Build history of the part. All positions in model axes, mm. Round coordinates to 2 decimals unless told otherwise and drop trailing zeros. Write each loop counter-clockwise with the first axis right and the second up, starting at its lowest first coordinate (ties: lowest second). Pieces come first, ordered by that corner, then holes.
from build123d import *

# Parameters (mm, degrees)
BOSS_EXTRUDE1_DEPTH = 14
CHAMFER1_SIZE       = 2


with BuildPart() as part:
    # Sketch1 → Boss-Extrude1 (new body)
    with BuildSketch(Plane.XY):
        Polygon((4, 3), (61, 3), (53, 31), (12, 38), align=None)
    extrude(amount=BOSS_EXTRUDE1_DEPTH)

    # Chamfer1
    chamfer1_edges = [part.edges().sort_by_distance(p)[0] for p in [
        (53, 31, 7),
    ]]
    chamfer(chamfer1_edges, length=CHAMFER1_SIZE)


solid = part.part
1) Wall check: L1, parallel to X at y = 11, z = 2.25; L2, parallel to X at y = 15.5, z = 2; L3, parallel to Y at x = 33, z = 4. Give the ranges that are in metal, low to high.
Results:
L1: x = 5.83 to 58.71
L2: x = 6.86 to 57.43
L3: y = 3 to 34.41
2) Slice it at C-C (y = 11). Write the cut outline in (x, z), plus the area to 3 significant figures.
Results:
outline: (5.83, 0) - (58.71, 0) - (58.71, 14) - (5.83, 14) - close
area: 740 mm2
3) Slice it at A-A (z = 6). Write the cut outline in (x, y).
Results:
outline: (4, 3) - (61, 3) - (53.55, 29.08) - (51.03, 31.34) - (12, 38) - close
4) Slice it at B-B (x = 8). Write the cut outline in (y, z), plus the area to 3 significant figures.
Results:
outline: (3, 0) - (20.5, 0) - (20.5, 14) - (3, 14) - close
area: 245 mm2
5) Pin check, flat tip, straight feed: pin 1 Ø1.5 at (y, z) = (24.5, 10) entering from -X. Stop position of the tip, or through.
Results:
pin 1: stops at x = 8.74
